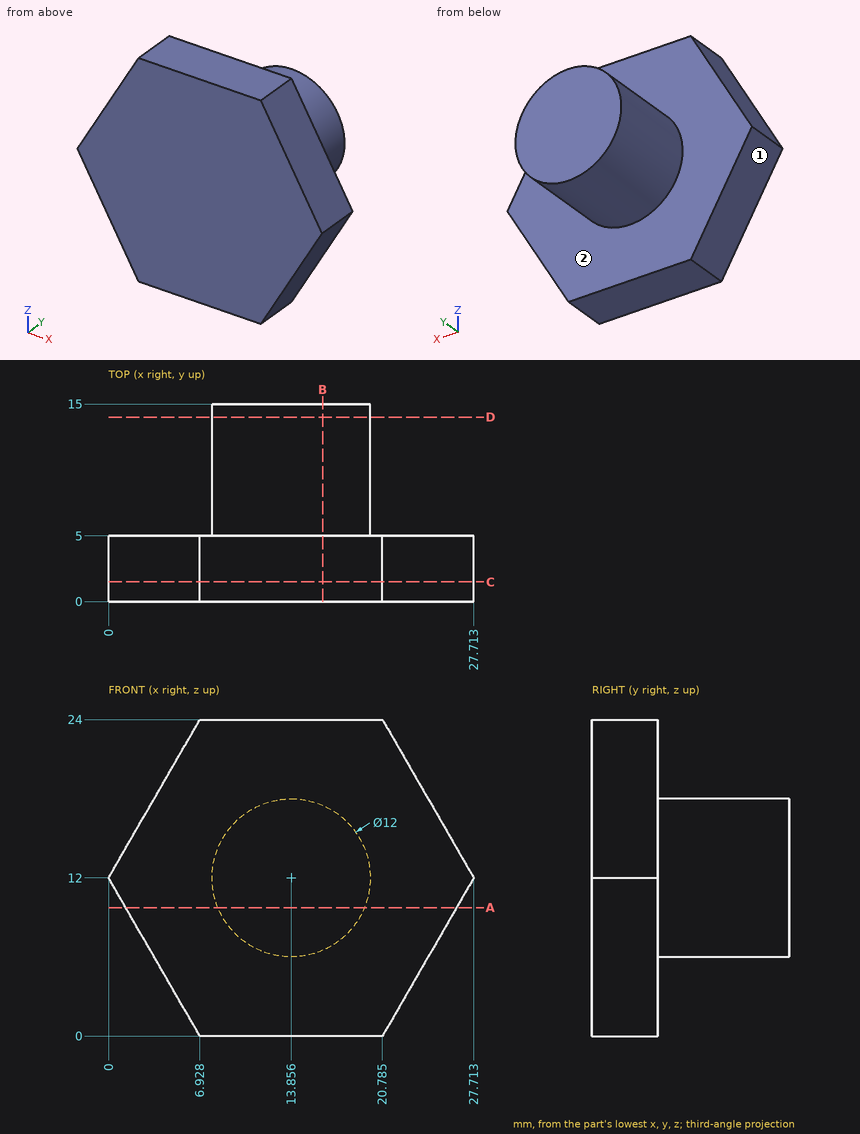
Study the drawing (mm; zero at the part's minimum x, y, z) and answer. A direction names the side the tool comes from. Coordinates: 2 decimals unless noted, no trailing zeros. Write each loop counter-clockwise with the first axis right and the second up, starting at its lowest first coordinate (ties: lowest second). Pieces come first, ordered by that corner, then holes. Notation, with made-up numbers: (-36, -22) -> (2, -22) arc R23 ccw to (2, 16) -> close; hole circle Ø9 at (59, 17.5). An arc over 180 degrees is marked (long way). Write each question's results on one line, items separated by ' | '. Start each with the question number.
1) A tool of negligible diameter and unlimited length cuts with its end or side. For the marked faces 1 and 2, from which of +Z, -Z, +X, -X, +Y, -Y can it reach the whole face along a straight path? Write none if from no direction.
2) A cutting plane is placed at B-B (x = 16.25). Determine the outline of the cut face in (y, z).
3) Straight lines are drawn through the part: probe 1 along Y at (x, z) = (7.5, 19.25); probe 2 along X at (y, z) = (12, 12); probe 3 along Z at (x, y) = (15.25, 11) (1 decimal). For each, find the intervals that lie inside material, in ascending order.
4) A cutting plane is placed at C-C (y = 1.5). Determine the outline of the cut face in (x, z) (1 decimal), then the cut area to 3 significant figures.
5) Flat-ended cylindrical pins translate along their axes: pin 1 Ø1 at (x, y) = (5, 2.5) entering from +Z (1 decimal); pin 2 Ø1.5 at (y, z) = (3.5, 4) entering from +X; pin 3 Ø8 at (y, z) = (11, 17.5) entering from -X. Find the tip coordinate at first contact, or state that the pin passes through.
6) A cutting plane is placed at D-D (y = 14). Determine the outline of the cut face in (x, z).
7) A cutting plane is placed at A-A (z = 9.75). Determine the outline of the cut face in (x, y) (1 decimal).
Values follow:
1) face 1: -Z, -X, +Y, -Y | face 2: +Y
2) outline: (0, 0) -> (5, 0) -> (5, 6.5) -> (15, 6.5) -> (15, 17.5) -> (5, 17.5) -> (5, 24) -> (0, 24) -> close
3) probe 1: 0 to 5 | probe 2: 7.86 to 19.86 | probe 3: 6.2 to 17.8
4) outline: (0, 12) -> (6.9, 0) -> (20.8, 0) -> (27.7, 12) -> (20.8, 24) -> (6.9, 24) -> close | area: 499 mm²
5) pin 1: z = 21.5 | pin 2: x = 23.53 | pin 3: x = 8.05
6) outline: circle Ø12 at (13.86, 12)
7) outline: (1.3, 0) -> (26.4, 0) -> (26.4, 5) -> (19.4, 5) -> (19.4, 15) -> (8.3, 15) -> (8.3, 5) -> (1.3, 5) -> close
